The model under review builds one solid part; all positions refer to its coordinate system, in mm. A direction names the side the tool comes from. Coordinates: 2 decimals unless noted, no trailing zeros. Loops run counter-clockwise (first coordinate to the right, second up) from the corner with the lowest first, then second, coordinate; pieces in that order, holes last. Notation, with made-up numbers: (13, 50) -> (18, 50) arc R18 cw to (18, 80) -> close; hole circle Ø9 at (-2.75, 15.25). An arc over 180 degrees is marked (long way). One line per question, with ' | ' between items. Start each with the question number.
from build123d import *

# Parameters (mm, degrees)
F0_R          = 1.76
F1_DEPTH      = 8.6
F1_DEPTH_BACK = 8.6
F2_R          = 5.9
F3_DEPTH      = 3.52
F4_R          = 4.225
F5_DEPTH      = 5


with BuildPart() as f1:
    # F0 (on Right) → F1 (new body, two sides)
    with BuildSketch(Plane.YZ) as f1_sk:
        with Locations((0, 1.76)):
            Circle(F0_R)
    extrude(amount=F1_DEPTH)
    extrude(f1_sk.sketch, amount=-F1_DEPTH_BACK)

    # F2 (on Top) → F3 (join)
    with BuildSketch(Plane.XY):
        Circle(F2_R)
    extrude(amount=F3_DEPTH)

    # F4 (on face) → F5 (cut)
    with BuildSketch(Plane.XY.offset(3.52)):
        Circle(F4_R)
    extrude(amount=-F5_DEPTH, mode=Mode.SUBTRACT)


solid = f1.part
1) Consider section C-C, the plane z = 1.76. Write out the cut boundary in (x, y) (3 decimals).
2) Mouldability with a two-part tool opening along Y and no side actions: class faces 3 (the face through (4.03, 1.27, 1.78)), 4 (the face through (7.14, -1.76, 1.84)), 5 (the face through (0.1, 5.9, 1.7)) as +Y half, -Y half, draft (parallel to the pull), parting line (faces both ways), or undercut.
3) Insertion check: pin 1 Ø2 at (y, z) = (4, 2) entering from -X; pin 2 Ø2 at (y, z) = (3.5, 1) entering from -X. Each pin has a flat end and moves straight along its axis. Give the tip position at first contact, or say it passes through.
4) Wall thickness on L1, parallel to Y at x = 0, z = 2.05 (3 decimals); L2, parallel to X at y = 3.75, z = 2.25; L3, parallel to Y at x = 3, z = 0.4 (3 decimals): over which ranges is each line inside the solid? List them lowest first.
5) Consider section D-D, the plane z = 0.5. Write out the cut boundary in (x, y) (3 decimals), plus the area to 3 significant figures.
6) Consider section A-A, the plane x = 0. Write out the cut boundary in (y, z) (3 decimals).
7) Consider section B-B, the plane y = -4. Write out the cut boundary in (x, z), plus the area to 3 significant figures.
8) Machinability: for faces 1 (the face through (3, -4, 3.52)), 2 (the face through (-7.09, -1.76, 1.84)), which of the approach directions +Z, -Z, +X, -X, +Y, -Y give a long, thin tool a straight path to every point of the face, cutting with its end or side? Answer none if there is none.
Filled sheet:
1) outline: (-8.6, -1.76) -> (-5.631, -1.76) arc R5.9 ccw to (5.631, -1.76) -> (8.6, -1.76) -> (8.6, 1.76) -> (5.631, 1.76) arc R5.9 ccw to (-5.631, 1.76) -> (-8.6, 1.76) -> close; hole circle Ø8.45 at (0, 0)
2) face 3: undercut | face 4: parting line | face 5: +Y half
3) pin 1: x = -5.08 | pin 2: x = -5.34
4) L1: -5.9 to -4.225, 4.225 to 5.9 | L2: -4.55 to -1.95, 1.95 to 4.55 | L3: -5.08 to -2.975, 2.975 to 5.08
5) outline: (-8.6, -1.229) -> (-5.771, -1.229) arc R5.9 ccw to (5.771, -1.229) -> (8.6, -1.229) -> (8.6, 1.229) -> (5.771, 1.229) arc R5.9 ccw to (-5.771, 1.229) -> (-8.6, 1.229) -> close; hole circle Ø8.45 at (0, 0) | area: 66.8 mm^2
6) outline: (-5.9, 0) -> (-4.225, 0) -> (-4.225, 3.52) -> (-5.9, 3.52) -> close; (4.225, 0) -> (5.9, 0) -> (5.9, 3.52) -> (4.225, 3.52) -> close
7) outline: (-4.34, 0) -> (-1.36, 0) -> (-1.36, 3.52) -> (-4.34, 3.52) -> close; (1.36, 0) -> (4.34, 0) -> (4.34, 3.52) -> (1.36, 3.52) -> close | area: 21.0 mm^2
8) face 1: +Z, +X, -X, +Y, -Y | face 2: -X
